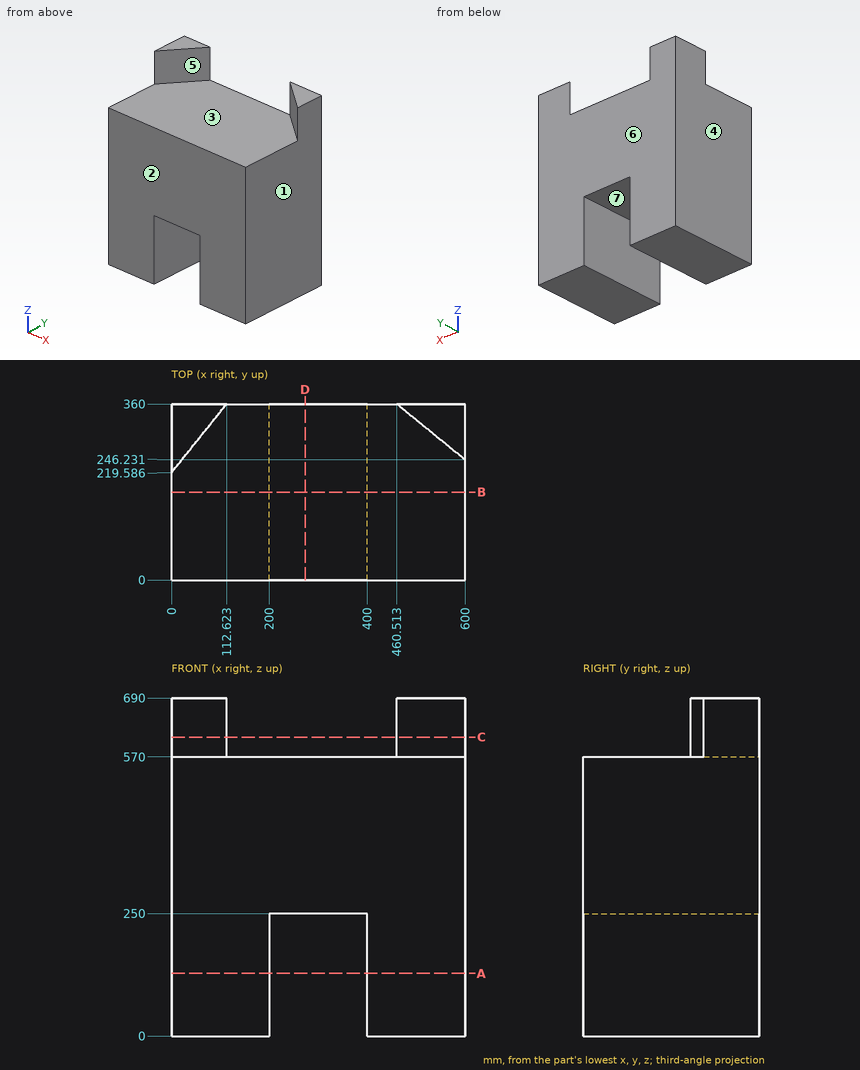
The figure shows three views and two pictorial views of one solid part (mm, origin at its lowest corner). Answer the questions. A direction names the side the tool comes from. Give positions to 0.01 mm unless a question says otherwise; leave off trailing zeros. Write each loop counter-clockwise with the first axis right and the second up, starting at its lowest first coordinate (ties: lowest second). Pieces come first, ordered by that corner, then holes. Notation, with made-up numbers: (38, -4) - (48, -4) arc R21 ccw to (48, 16) - close; hole circle Ø10 at (-15, 74.5). An arc over 180 degrees is marked (long way). Use one line per item in the form item = value. Start each with the question number.
1) Find section A-A on z = 128. Determine the outline of the cut face in (x, y), plus the area to 3 significant figures.
2) The mould has two halves that part along X. Classify the marked faces 1, 2, 3 and 4: pulls with the +X half, pulls with the -X half, needs draft (parallel to the pull), parting line crosses it, or undercut.
3) Find section D-D on x = 273. Determine the outline of the cut face in (y, z), plus the area to 3 significant figures.
4) Consider line 1 along X through (y, z) = (204.5, 37); line 2 along Z through (x, y) = (423.5, 19); line 3 along Z through (x, y) = (393, 270.5). Determine where each line is inside the solid, lowest interval first. Write a range as from..to.
5) A tool of negligible diameter and unlimited length cuts with its end or side. For the marked faces 5, 6 and 7, from which of +Z, -Z, +X, -X, +Y, -Y can it reach the whole face along a straight path? Write none if from no direction.
6) Find section B-B on y = 180. Determine the outline of the cut face in (x, z), plus the area to 3 significant figures.
7) Find section C-C on z = 610.5. Determine the outline of the cut face in (x, y).
8) A flat-ended cylindrical pin translates along its axis: pin 1 Ø6 at (x, y) = (375.5, 230) entering from -Z. Find the tip coordinate at first contact, or state that the pin passes through.
Geometry results:
q1.outline = (0, 0) - (200, 0) - (200, 360) - (0, 360) - close; (400, 0) - (600, 0) - (600, 360) - (400, 360) - close
q1.area = 144,000 mm2
q2.face_1 = pulls with the +X half
q2.face_2 = needs draft
q2.face_3 = undercut
q2.face_4 = pulls with the -X half
q3.outline = (0, 250) - (360, 250) - (360, 570) - (0, 570) - close
q3.area = 115,000 mm2
q4.line_1 = 0..200, 400..600
q4.line_2 = 0..570
q4.line_3 = 250..570
q5.face_5 = +Z, -Y
q5.face_6 = +Z, -Z, +X, -X, +Y
q5.face_7 = -Z, +Y, -Y
q6.outline = (0, 0) - (200, 0) - (200, 250) - (400, 250) - (400, 0) - (600, 0) - (600, 570) - (0, 570) - close
q6.area = 292,000 mm2
q7.outline = (0, 219.59) - (112.62, 360) - (0, 360) - close; (460.51, 360) - (600, 246.23) - (600, 360) - close
q8.pin_1 = 250
